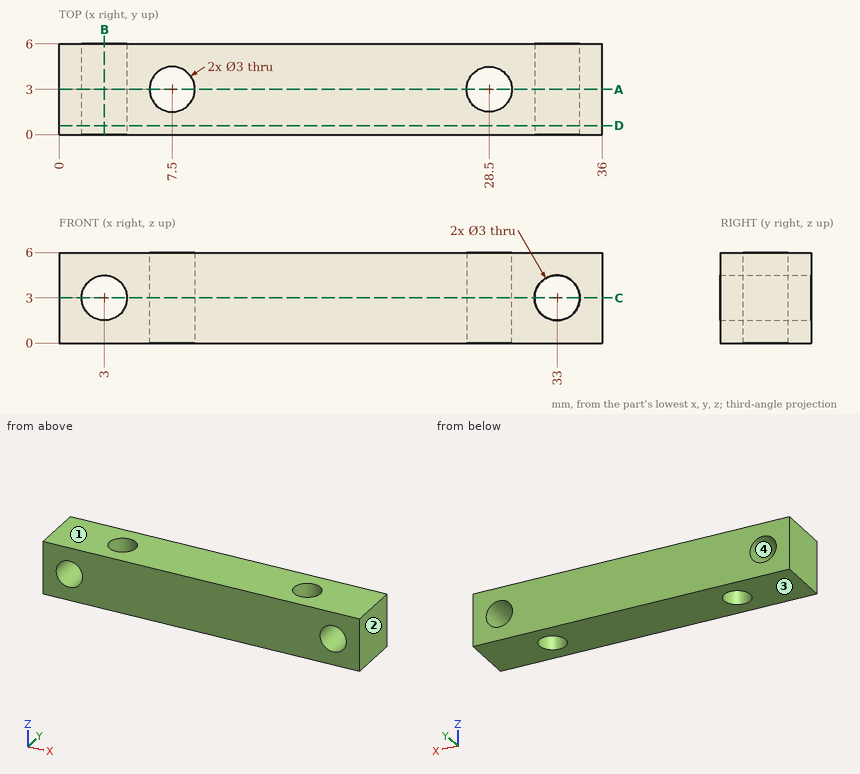
Answer from the drawing. Dimensions are ordinates in mm from the lowest x, y and z of the part. Give positions to 0.01 mm unless a question says otherwise; leave off trailing zeros. Loops run counter-clockwise (first coordinate to the right, second up) from the corner with the lowest first, then second, coordinate; pieces in that order, holes last.
Item 1: The part is cut by section A-A (y = 3). Write down the section's boundary in (x, z), and give its area (3 significant figures).
Item 2: Find the intervals of material crossed by line 1 along X through (y, z) = (5.5, 4.1); line 2 along Y through (x, z) = (7.5, 1.6); line 3 along X through (y, z) = (4.35, 5.5), in increasing order.
Item 3: The part is cut by section D-D (y = 0.6). Write down the section's boundary in (x, z).
Item 4: The part is cut by section C-C (z = 3). Write down the section's boundary in (x, y), and give its area (3 significant figures).
Item 5: The mould has two halves that part along Z. Classify the marked faces 1, 2, 3 and 4: released by +Z, released by -Z, zero draft, split by the parting line, or undercut.
Item 6: The part is cut by section B-B (x = 3). Write down the section's boundary in (y, z), and give its area (3 significant figures).
Taken from the geometry:
1. outline: (0, 0) - (6, 0) - (6, 6) - (0, 6) - close; (9, 0) - (27, 0) - (27, 6) - (9, 6) - close; (30, 0) - (36, 0) - (36, 6) - (30, 6) - close; hole circle Ø3 at (3, 3); hole circle Ø3 at (33, 3)
1. area: 166 mm2
2. line 1: x = 0 to 1.98, 4.02 to 31.98, 34.02 to 36
2. line 2: y = 0 to 1.5, 4.5 to 6
2. line 3: x = 0 to 6.85, 8.15 to 27.85, 29.15 to 36
3. outline: (0, 0) - (36, 0) - (36, 6) - (0, 6) - close; hole circle Ø3 at (3, 3); hole circle Ø3 at (33, 3)
4. outline: (0, 0) - (1.5, 0) - (1.5, 6) - (0, 6) - close; (4.5, 0) - (31.5, 0) - (31.5, 6) - (4.5, 6) - close; (34.5, 0) - (36, 0) - (36, 6) - (34.5, 6) - close; hole circle Ø3 at (7.5, 3); hole circle Ø3 at (28.5, 3)
4. area: 166 mm2
5. face 1: released by +Z
5. face 2: zero draft
5. face 3: released by -Z
5. face 4: undercut
6. outline: (0, 0) - (6, 0) - (6, 1.5) - (0, 1.5) - close; (0, 4.5) - (6, 4.5) - (6, 6) - (0, 6) - close
6. area: 18.0 mm2
